Read the model definition and answer for the solid it produces. Units are mm, in the model's axes. Give positions to 0.01 mm unless a question says otherwise; leave off trailing zeros. Write each loop counter-clockwise with the first axis right and the second up, starting at its lowest first coordinate (ties: lowest second). Pieces come first, ordered by that corner, then holes. Notation, with made-up numbers: M 9,74.25 L 17,74.25 A19 ccw 17,81.25 Z; hole C -29,20.25 d11. An arc over 180 degrees is marked long. Answer as CSV lines item,"result". Start each with the question number.
```python
from build123d import *

# Parameters (mm, degrees)
F1_DEPTH = 6
F2_R     = 5
F3_R     = 2
F4_R     = 0.25


with BuildPart() as f1:
    # F0 (on Top) → F1 (new body)
    with BuildSketch(Plane.XY):
        with BuildLine():
            Line((-11.8683932183, 4), (-15.5, 4))
            Line((-15.5, 4), (-15.5, -4))
            Line((-15.5, -4), (15.5, -4))
            Line((15.5, -4), (15.5, 4))
            Line((15.5, 4), (11.8683932183, 4))
            ThreePointArc((11.8683932183, 4), (12.9517769752, 2.9530277574), (13.35, 1.5))
            ThreePointArc((13.35, 1.5), (9.0469722426, -0.9517769752), (9.1316067817, 4))
            Line((9.1316067817, 4), (-9.1316067817, 4))
            ThreePointArc((-9.1316067817, 4), (-8.0482230248, 2.9530277574), (-7.65, 1.5))
            ThreePointArc((-7.65, 1.5), (-11.9530277574, -0.9517769752), (-11.8683932183, 4))
        make_face()
    extrude(amount=F1_DEPTH)

    # F2
    f2_edges = [f1.edges().sort_by_distance(p)[0] for p in [
        (15.5, -4, 3),
        (-15.5, -4, 3),
    ]]
    fillet(f2_edges, radius=F2_R)

    # F3
    f3_edges = [f1.edges().sort_by_distance(p)[0] for p in [
        (-15.5, 4, 3),
        (15.5, 4, 3),
    ]]
    fillet(f3_edges, radius=F3_R)

    # F4
    f4_edges = [f1.edges().sort_by_distance(p)[0] for p in [
        (9.131607, 4, 3),
        (11.868393, 4, 3),
        (-9.131607, 4, 3),
        (-11.868393, 4, 3),
    ]]
    fillet(f4_edges, radius=F4_R)


solid = f1.part
```
1. Find section B-B on z = 2.75. Determine the outline of the cut face in (x, y).
2. Determine the mould class of faces 1 (the face through (-15.5, 1.5, 3)), 2 (the face through (0, 0, 0)), 3 (the face through (0, 0, 6)) for opening direction Z: +Z half, -Z half, draft (parallel to the pull), parting line (faces both ways), or undercut.
3. Find section D-D on y = 3. Determine the outline of the cut face in (x, z), then the cut area to 3 significant figures.
4. Given pin 1 (4.5 mm diameter, centred on x = 10.5, y = 1.5, fed in from +Z), flat-ended and moving along its own axis, determine where the tip first touches the part or whether it passes through.
5. Find section A-A on y = -1. Determine the outline of the cut face in (x, z).
6. Find the intervals of material crossed by line 1 (X direction, y = 1.5, z = 1.4); line 2 (X direction, y = 2.5, z = 2.25); line 3 (Y direction, x = 10.5, z = 1.9), in increasing order. Write a range as [from, to].
7. Find section C-C on y = -3. Determine the outline of the cut face in (x, z).
Computed:
1,outline,"M -15.5,1 A5 ccw -10.5,-4 L 10.5,-4 A5 ccw 15.5,1 L 15.5,2 A2 ccw 13.5,4 L 12.63,4 A0.25 ccw 12.46,3.57 A2.85 cw long 8.54,3.57 A0.25 ccw 8.37,4 L -8.37,4 A0.25 ccw -8.54,3.57 A2.85 cw long -12.46,3.57 A0.25 ccw -12.63,4 L -13.5,4 A2 ccw -15.5,2 Z"
2,face 1,"draft"
2,face 2,"-Z half"
2,face 3,"+Z half"
3,outline,"M -15.23,0 L -12.92,0 L -12.92,6 L -15.23,6 Z; M -8.08,0 L 8.08,0 L 8.08,6 L -8.08,6 Z; M 12.92,0 L 15.23,0 L 15.23,6 L 12.92,6 Z"
3,area,"125 mm^2"
4,pin 1,"passes through"
5,outline,"M -15.08,0 L -11.87,0 L -11.87,6 L -15.08,6 Z; M -9.13,0 L 9.13,0 L 9.13,6 L -9.13,6 Z; M 11.87,0 L 15.08,0 L 15.08,6 L 11.87,6 Z"
6,line 1,"x = [-15.5, -13.35], [-7.65, 7.65], [13.35, 15.5]"
6,line 2,"x = [-15.44, -13.17], [-7.83, 7.83], [13.17, 15.44]"
6,line 3,"y = [-4, -1.35]"
7,outline,"M -13.5,0 L 13.5,0 L 13.5,6 L -13.5,6 Z"
